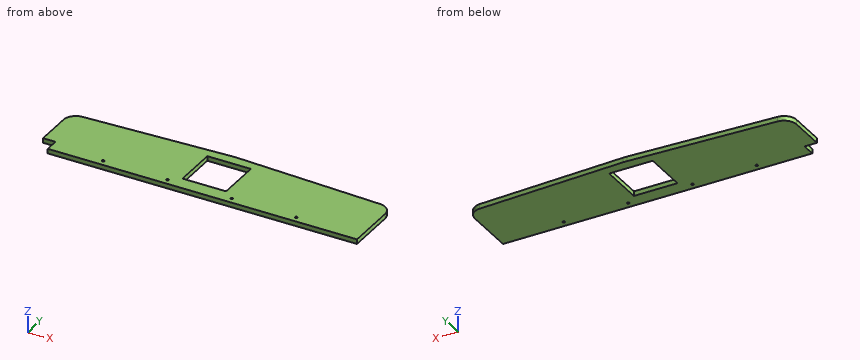
from build123d import *

# Parameters (mm, degrees)
BOSS_EXTRUDE1_DEPTH         = 4.7625
FILLET1_R                   = 25.4
FILLET2_R                   = 101.6
SKETCH3_W                   = 25.4
SKETCH3_H                   = 27.686
CUT_EXTRUDE1_DEPTH          = 370.281286979
SKETCH5_W                   = 88.9
SKETCH5_H                   = 88.9
CUT_EXTRUDE2_DEPTH          = 370.281286979
TAP_DRILL_FOR_M6X1_0_TAP1_D = 5


with BuildPart() as part:
    # Sketch2 → Boss-Extrude1 (new, symmetric)
    with BuildSketch(Plane.XY):
        Polygon((-328.331514278, 55.6895), (-328.331514278, 154.489500012), (0, 168.8465), (328.285794278, 154.489500012), (328.285794278, 55.6895), (328.285794278, 29.289499968), (-328.331514278, 29.289499968), align=None)
    extrude(amount=BOSS_EXTRUDE1_DEPTH, both=True)

    # Fillet1
    fillet1_edges = [part.edges().sort_by_distance(p)[0] for p in [
        (-328.331514278, 154.489500012, 0),
        (328.285794278, 154.489500012, 0),
    ]]
    fillet(fillet1_edges, radius=FILLET1_R)

    # Fillet2
    # the kernel refuses this fillet: 101.6 mm, written as the material it takes off along each edge
    with BuildSketch(Plane(origin=(0, 168.8465, 15.869968436), x_dir=(-0.9990453371749675, -0.04368540109642698, 0), z_dir=(0, 0, -1))) as fillet2_piece_1:
        with BuildLine():
            CenterArc((FILLET2_R * 0.0437301906922, -FILLET2_R), FILLET2_R, 90, 5.00792009)
            Line((-FILLET2_R * 0.0435632568505, -FILLET2_R * 0.00381735910722), (0, 0))
            Line((0, 0), (FILLET2_R * 0.0437301906922, 0))
        make_face()
    extrude(amount=31.739936872, mode=Mode.SUBTRACT)

    # Sketch3 → Cut-Extrude1 (cut, through all)
    with BuildSketch(Plane.XY.offset(4.7625)):
        with Locations((-315.631514278, 43.132499968)):
            Rectangle(SKETCH3_W, SKETCH3_H)
    extrude(amount=-CUT_EXTRUDE1_DEPTH, mode=Mode.SUBTRACT)

    # Sketch5 → Cut-Extrude2 (cut, through all)
    with BuildSketch(Plane.XY.offset(4.7625)):
        with Locations((0.067349574, 102.81865045)):
            Rectangle(SKETCH5_W, SKETCH5_H)
    extrude(amount=-CUT_EXTRUDE2_DEPTH, mode=Mode.SUBTRACT)

    # Tap Drill for M6x1.0 Tap1 (through all)
    with Locations(Plane.XY.offset(4.7625)):
        with Locations((-197.013514278, 41.989499968), (-65.695514278, 41.989499968), (65.622485722, 41.989499968), (196.940485722, 41.989499968)):
            Hole(TAP_DRILL_FOR_M6X1_0_TAP1_D / 2)


solid = part.part
The model under review builds one solid part; all positions refer to its coordinate system, in mm. Give positions to 0.01 mm unless a question says otherwise; leave off trailing zeros. Order: outer loops, then holes, each group sorted by start corner. A loop starts at its lowest first (then second) coordinate and runs counter-clockwise, first axis right, second up. Notation, with made-up numbers: M -6.75,17 L 48.25,17 A25 ccw 48.25,42 Z; hole C 45,-15.5 d10. An arc over 180 degrees is marked long. Answer in a Markdown table with one row per item. Add a question column.
1. To check wall thickness, follow line 1 along X through (y, z) = (118, 1.5); line 2 along X through (y, z) = (40, -1.25); line 3 along Y through (x, z) = (-9, 3.75). State the ranges of each line that lie inside material, in increasing order.
2. Add section B-B on x = 37. State the section outline as (y, z) points, plus the area to 3 significant figures.
3. Add section C-C on z = 1.5. State the section outline as (x, y) points, plus the area to 3 significant figures.
4. Add section A-A on y = 99. State the section outline as (x, z) points.
5. For pin 1 Ø5 at (y, z) = (40, 2) entering from -X; pin 2 Ø3 at (x, y) = (65.62, 41.99) entering from -Z; pin 3 Ø2 at (y, z) = (141, -3.5) entering from +X; pin 4 Ø4 at (x, z) = (178.5, 2) entering from +Y, all flat-tipped, find the tip position at first contact; note any pin that passes through.
6. Add section D-D on x = 239. State the section outline as (y, z) points, plus the area to 3 significant figures.
The answers:
| question | item | result |
|---|---|---|
| 1 | line 1 | -328.33 to -44.38, 44.52 to 328.29 |
| 1 | line 2 | -302.93 to -198.53, -195.5 to -67.21, -64.18 to 64.11, 67.14 to 195.43, 198.45 to 328.29 |
| 1 | line 3 | 29.29 to 58.37, 147.27 to 168.45 |
| 2 | outline | M 29.29,-4.76 L 58.37,-4.76 L 58.37,4.76 L 29.29,4.76 Z; M 147.27,-4.76 L 167.23,-4.76 L 167.23,4.76 L 147.27,4.76 Z |
| 2 | area | 467 mm2 |
| 3 | outline | M -328.33,56.98 L -302.93,56.98 L -302.93,29.29 L 328.29,29.29 L 328.29,130.18 A25.4 ccw 304,155.55 L 4.44,168.65 A101.6 ccw -4.44,168.65 L -304.04,155.55 A25.4 ccw -328.33,130.18 Z; hole C -197.01,41.99 d5; hole C -65.7,41.99 d5; hole M -44.38,58.37 L 44.52,58.37 L 44.52,147.27 L -44.38,147.27 Z; hole C 65.62,41.99 d5; hole C 196.94,41.99 d5 |
| 3 | area | 78,000 mm2 |
| 4 | outline | M -328.33,-4.76 L -44.38,-4.76 L -44.38,4.76 L -328.33,4.76 Z; M 44.52,-4.76 L 328.29,-4.76 L 328.29,4.76 L 44.52,4.76 Z |
| 5 | pin 1 | x = -302.93 |
| 5 | pin 2 | through |
| 5 | pin 3 | x = 326.31 |
| 5 | pin 4 | y = 161.13 |
| 6 | outline | M 29.29,-4.76 L 158.39,-4.76 L 158.39,4.76 L 29.29,4.76 Z |
| 6 | area | 1,230 mm2 |
